Here's the drawing with two shaded views (mm, measured from the low corner). I have some questions. A direction names the side the tool comes from. Give positions to 0.01 mm unless a question says otherwise; leave off trailing zeros. Order: outer loops, then holes, each group sorted by start corner. A loop starts at its lowest first (then second) coordinate and runs counter-clockwise, first axis right, second up. Notation, with made-up numbers: M 52.5,57.5 L 108.5,57.5 A15 cw 108.5,62.5 Z; hole C -20.75,37 d7. An arc over 180 degrees is marked long. Write each question's results on one line, items separated by ' | '.
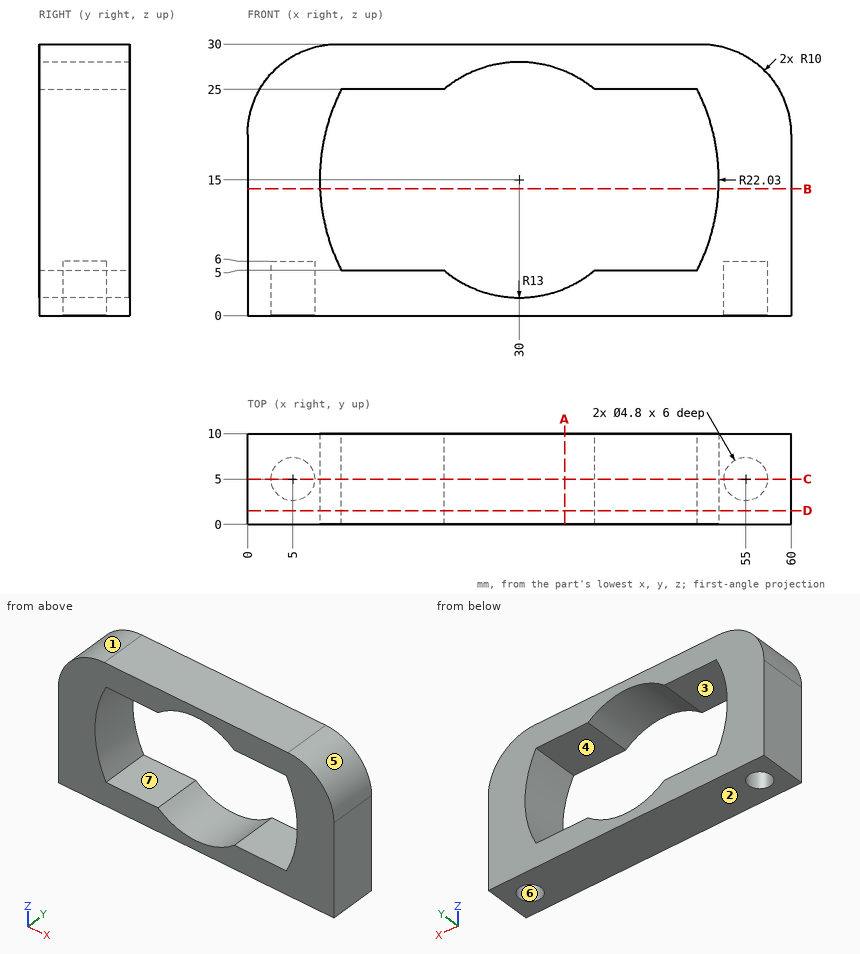
(1) Will these pins go through, and if not, where does the flat tip stop? P1, Ø2.5, axis at x = 55, y = 5.5, coming from the -Z side; P2, Ø4.5, axis at x = 5, y = 5, coming from the +Z side.
Data:
P1: stops at z = 6 | P2: stops at z = 29.61
(2) For the marked faces 5, 6 and 7, which set-ups out of +Z, -Z, +X, -X, +Y, -Y let a thin tool reach every point of the face, with its end or its side?
Data:
face 5: +Z, +X, +Y, -Y | face 6: -Z | face 7: +Y, -Y
(3) Imagine slicing it at B-B, the plane z = 14. Write out the boundary of the cut face in (x, y), plus the area to 3 significant figures.
Data:
outline: M 0,0 L 7.99,0 L 7.99,10 L 0,10 Z; M 52.01,0 L 60,0 L 60,10 L 52.01,10 Z | area: 160 mm2
(4) Imagine slicing it at A-A, the plane x = 35. Write out the boundary of the cut face in (y, z), plus the area to 3 significant figures.
Data:
outline: M 0,0 L 10,0 L 10,3 L 0,3 Z; M 0,27 L 10,27 L 10,30 L 0,30 Z | area: 60.0 mm2
(5) Imagine slicing it at D-D, the plane y = 1.5. Write out the boundary of the cut face in (x, z).
Data:
outline: M 0,0 L 60,0 L 60,20 A10 ccw 50,30 L 10,30 A10 ccw 0,20 Z; hole M 10.37,5 L 21.69,5 A13 ccw 38.31,5 L 49.63,5 A22.03 ccw 49.63,25 L 38.31,25 A13 ccw 21.69,25 L 10.37,25 A22.03 ccw Z
(6) We'd pull the mould along X, two halves only. Please class the marked faces 1, 2, 3 and 4: +X half, -X half, draft (parallel to the pull), parting line (faces both ways), or undercut.
Data:
face 1: -X half | face 2: draft | face 3: undercut | face 4: undercut
(7) Imagine slicing it at C-C, the plane y = 5. Write out the boundary of the cut face in (x, z).
Data:
outline: M 0,0 L 2.6,0 L 2.6,6 L 7.4,6 L 7.4,0 L 52.6,0 L 52.6,6 L 57.4,6 L 57.4,0 L 60,0 L 60,20 A10 ccw 50,30 L 10,30 A10 ccw 0,20 Z; hole M 10.37,5 L 21.69,5 A13 ccw 38.31,5 L 49.63,5 A22.03 ccw 49.63,25 L 38.31,25 A13 ccw 21.69,25 L 10.37,25 A22.03 ccw Z
(8) I need wall thicknesses on L1, parallel to Z at x = 11.5, y = 3.5; L2, parallel to Y at x = 55, z = 4.2; L3, parallel to X at y = 4, z = 7.5. Which ranges of each line are inside material? Lowest first, please. Write a range as from..to.
Data:
L1: z = 0..5, 25..30 | L2: y = 0..2.6, 7.4..10 | L3: x = 0..9.29, 50.71..60
